Part model, mm, in its own coordinate system. Give positions to 0.01 mm unless a question says otherwise; leave off trailing zeros. Order: outer loops, then holes, each group sorted by start corner. A loop starts at its lowest first (then second) coordinate and runs counter-clockwise, first axis right, second up. Notation, with made-up numbers: (70, 88.25) - (80, 88.25) arc R17 cw to (80, 113.25) - close; hole circle Ø2 at (84.25, 2.25). An arc over 180 degrees is marked (long way). One line per item, written item: value.
```python
from build123d import *

# Parameters (mm, degrees)
SKETCH1_R           = 7.439633922
BOSS_EXTRUDE1_DEPTH = 10


with BuildPart() as part:
    # Sketch1 → Boss-Extrude1 (new body)
    with BuildSketch(Plane.XY):
        with BuildLine():
            Line((333.85321321, 48.612982521), (353.85321321, 48.612982521))
            ThreePointArc((353.85321321, 48.612982521), (368.85321321, 33.612982521), (353.85321321, 18.612982521))
            Line((353.85321321, 18.612982521), (333.85321321, 18.612982521))
            Line((333.85321321, 18.612982521), (333.85321321, 48.612982521))
        make_face()
        with Locations((353.85321321, 33.612982521)):
            Circle(SKETCH1_R, mode=Mode.SUBTRACT)
    extrude(amount=BOSS_EXTRUDE1_DEPTH)

    # Sketch2 → Revolve2 (revolve)
    with BuildSketch(Plane.XY, mode=Mode.PRIVATE) as revolve2_sk:
        Polygon((333.85321321, 48.612982521), (333.85321321, 52.993606974), (331.026376732, 52.993606974), (331.026376732, 50.74274425), (66.67110802, 50.74274425), (66.67110802, 42.299173429), (318.559263149, 42.299173429), (318.559263149, 33.612982521), (333.85321321, 33.612982521), align=None)
    revolve(revolve2_sk.sketch.rotate(Axis((318.559263149, 33.612982521, 0), (1, 0, 0)), 90), axis=Axis((318.559263149, 33.612982521, 0), (1, 0, 0)))


solid = part.part
```
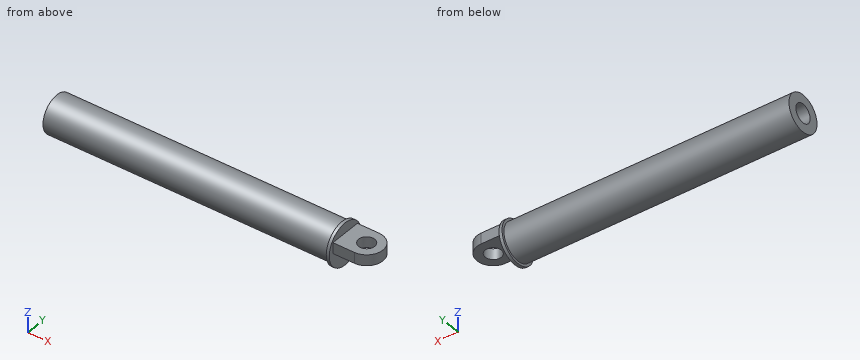
1) Drill centre lines: line 1 along X through (y, z) = (33.5, 6); line 2 along Y through (x, z) = (239, 0); line 3 along X through (y, z) = (43.5, -9). Where is each one in solid material? Low to high. Write a range as from..to.
Outcome:
line 1: x = 318.56..346.41, 361.29..368.85
line 2: y = 16.48..24.93, 42.3..50.74
line 3: x = 66.67..333.85
2) Cut at B-B, the plane z = -13. Give the cut face in (x, y), then the cut area to 3 significant figures.
Outcome:
outline: (66.67, 22.46) - (331.03, 22.46) - (331.03, 19.24) - (333.85, 19.24) - (333.85, 47.99) - (331.03, 47.99) - (331.03, 44.77) - (66.67, 44.77) - close
area: 5,980 mm^2
3) Cut at C-C, the plane x = 309.5. Give the cut face in (y, z).
Outcome:
outline: circle Ø34.26 at (33.61, 0); hole circle Ø17.37 at (33.61, 0)
4) Cut at A-A, the plane y = 30.5. Give the cut face in (x, z).
Outcome:
outline: (66.67, -16.84) - (331.03, -16.84) - (331.03, -19.13) - (333.85, -19.13) - (333.85, 0) - (347.1, 0) - (347.1, 10) - (333.85, 10) - (333.85, 19.13) - (331.03, 19.13) - (331.03, 16.84) - (66.67, 16.84) - (66.67, 8.11) - (318.56, 8.11) - (318.56, -8.11) - (66.67, -8.11) - close; (360.61, 0) - (368.53, 0) - (368.53, 10) - (360.61, 10) - close
5) Pin check, flat tips, straight feed: pin 1 (6 mm diameter, centred on x = 318.5, y = 38, fed in from -Z); pin 2 (1.5 mm diameter, centred on x = 213.5, z = -11, fed in from -Y); pin 3 (2 mm diameter, centred on x = 331, z = 9.5, fed in from +Y). Stop position of each tip, or through.
Outcome:
pin 1: stops at z = -17.07
pin 2: stops at y = 19.89
pin 3: stops at y = 51.03
